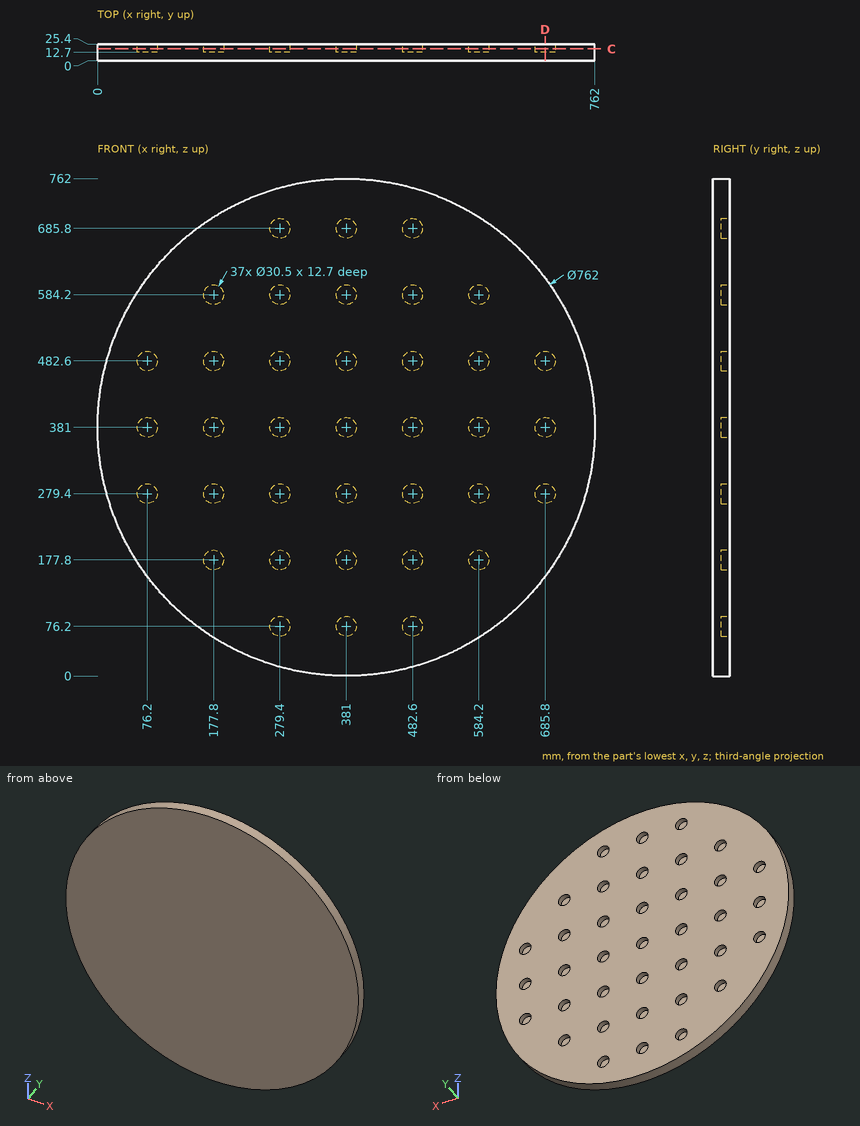
Answer from the drawing. Dimensions are ordinates in mm from the lowest x, y and z of the part. Coordinates: 2 decimals unless noted, no trailing zeros. Order: outer loops, then holes, each group sorted by start corner. A loop starts at its lowest first (then second) coordinate and runs counter-clockwise, first axis right, second up. Notation, with made-up numbers: M 4.5,-16 L 48.5,-16 A9 ccw 48.5,-1 Z; hole C -36,9 d1. An arc over 180 degrees is marked long. Put each result on its own line as item: value. Start each with the question number.
Item 1: Section C-C, the plane y = 18 is taken. Count the separate pieces of the cut face and the enclosed holes in it, plus the area to 3 significant figures.
Item 2: Section D-D, the plane x = 685.8 is taken. Determine the outline of the cut face in (y, z).
Item 3: Given pin 1 Ø18.5 at (x, z) = (279.4, 584.2) entering from +Y; pin 2 Ø12 at (x, y) = (571, 9.5) entering from +Z; pin 3 Ø8 at (x, y) = (615.5, 11.5) entering from +Z; pin 4 Ø5 at (x, z) = (308.5, 566) entering from -Y, each flat-ended and moving along its own axis, determine where each tip first touches the part or whether it passes through.
Item 4: Consider probe 1 along X at (y, z) = (22.5, 183.5); probe 2 along X at (y, z) = (21, 584.2); probe 3 along X at (y, z) = (18.5, 76.2). Determine where each line is inside the solid, lowest interval first. Write a range as [from, to].
Computed:
1. separate pieces: 1
1. enclosed holes: 37
1. area: 429,000 mm2
2. outline: M 0,152.4 L 25.4,152.4 L 25.4,264.15 L 12.7,264.15 L 12.7,294.65 L 25.4,294.65 L 25.4,365.75 L 12.7,365.75 L 12.7,396.25 L 25.4,396.25 L 25.4,467.35 L 12.7,467.35 L 12.7,497.85 L 25.4,497.85 L 25.4,609.6 L 0,609.6 Z
3. pin 1: stops at y = 12.7
3. pin 2: stops at z = 714.62
3. pin 3: stops at z = 684.37
3. pin 4: stops at y = 0
4. probe 1: x = [55.19, 163.66], [191.94, 265.26], [293.54, 366.86], [395.14, 468.46], [496.74, 570.06], [598.34, 706.81]
4. probe 2: x = [58.71, 162.55], [193.05, 264.15], [294.65, 365.75], [396.25, 467.35], [497.85, 568.95], [599.45, 703.29]
4. probe 3: x = [152.4, 264.15], [294.65, 365.75], [396.25, 467.35], [497.85, 609.6]
